Part model, mm, in its own coordinate system. Face numbers are marked on the shaded views. A direction names the side the tool comes from. Round coordinates to 2 decimals unless told otherwise and drop trailing zeros. Write each loop counter-clockwise with the first axis right and the second up, starting at its lowest first coordinate (ties: lowest second). Pieces come first, ordered by that corner, then holes.
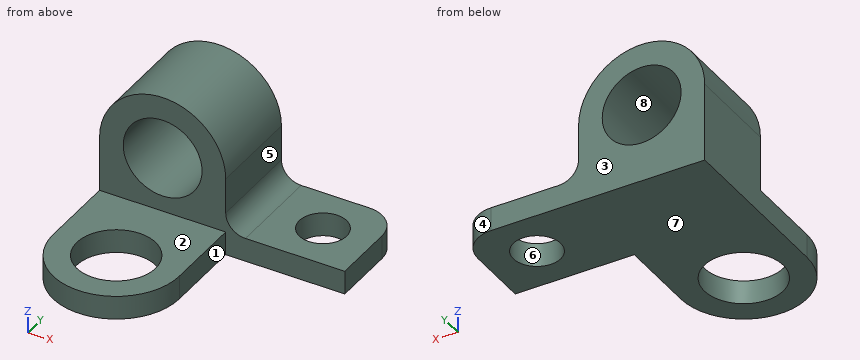
```python
from build123d import *

# Parameters (mm, degrees)
F0_R     = 50
F1_DEPTH = 120
F2_R     = 30
F3_DEPTH = 30
F4_R     = 50
F5_DEPTH = 30


with BuildPart() as f1:
    # F0 (on Front) → F1 (new body)
    with BuildSketch(Plane.XZ):
        with BuildLine():
            Line((0, 100), (0, 0))
            Line((0, 0), (311, 0))
            Line((311, 0), (311, 30))
            Line((311, 30), (185, 30))
            ThreePointArc((185, 30), (167.32233, 37.32233), (160, 55))
            Line((160, 55), (160, 100))
            ThreePointArc((160, 100), (80, 180), (0, 100))
        make_face()
        with Locations((80, 100)):
            Circle(F0_R, mode=Mode.SUBTRACT)
    extrude(amount=F1_DEPTH)

    # F2 (on face) → F3 (cut)
    with BuildSketch(Plane.XY.offset(30)):
        with Locations((248, -60)):
            Circle(F2_R)
        with BuildLine():
            Line((311, 0), (271, 0))
            ThreePointArc((271, 0), (299.284271, -11.715729), (311, -40))
            Line((311, -40), (311, 0))
        make_face()
    extrude(amount=-F3_DEPTH, mode=Mode.SUBTRACT)

    # F4 (on face) → F5 (join)
    with BuildSketch(Plane(origin=(0, 0, 0), x_dir=(1, 0, 0), z_dir=(0, 0, -1))):
        with BuildLine():
            Line((0, 220), (0, 120))
            Line((0, 120), (160, 120))
            Line((160, 120), (160, 220))
            ThreePointArc((160, 220), (80, 300), (0, 220))
        make_face()
        with Locations((80, 220)):
            Circle(F4_R, mode=Mode.SUBTRACT)
    extrude(amount=-F5_DEPTH)


solid = f1.part
```
Q1. Cut at B-B on x = 80. Write the cut outline in (y, z), plus the area to 3 significant figures.
Values follow:
outline: (-300, 0) - (-270, 0) - (-270, 30) - (-300, 30) - close; (-170, 0) - (0, 0) - (0, 50) - (-120, 50) - (-120, 30) - (-170, 30) - close; (-120, 150) - (0, 150) - (0, 180) - (-120, 180) - close
area: 12,000 mm2
Q2. Mould opens along Z. For the marked faces 6, 7 and 8 say: +Z half, -Z half, draft (parallel to the pull), parting line (faces both ways), or undercut.
Values follow:
face 6: draft
face 7: -Z half
face 8: undercut
Q3. Cut at A-A on y = -60. Write the cut outline in (x, z), plus the area to 3 significant figures.
Values follow:
outline: (0, 0) - (218, 0) - (218, 30) - (185, 30) arc R25 cw to (160, 55) - (160, 100) arc R80 ccw to (0, 100) - close; (278, 0) - (311, 0) - (311, 30) - (278, 30) - close; hole circle Ø100 at (80, 100)
area: 21,100 mm2
Q4. Drop flat-ended pins along their axis: pin 1 (10 mm diameter, centred on x = 220, y = -41, fed in from -Z); pin 2 (1.5 mm diameter, centred on y = -58.5, z = 90, fed in from +X); pin 3 (3 mm diameter, centred on x = 33, z = 63, fed in from -Y); pin 4 (6 mm diameter, centred on x = 81, y = -167, fed in from +Z). Give the stop position or say it passes through.
Values follow:
pin 1: stops at z = 0
pin 2: stops at x = 160
pin 3: stops at y = -120
pin 4: stops at z = 30
Q5. Cut at D-D on z = 134. Write the cut outline in (x, y).
Values follow:
outline: (7.58, -120) - (43.34, -120) - (43.34, 0) - (7.58, 0) - close; (116.66, -120) - (152.42, -120) - (152.42, 0) - (116.66, 0) - close
Q6. Cut at C-C on x = 248. Write the cut outline in (y, z), plus the area to 3 significant figures.
Values follow:
outline: (-120, 0) - (-90, 0) - (-90, 30) - (-120, 30) - close; (-30, 0) - (0, 0) - (0, 30) - (-30, 30) - close
area: 1,800 mm2
Q7. Which spindle directions (+Z, -Z, +X, -X, +Y, -Y) get a long thin tool onto all of the face, cutting with end or side? Do the marked faces 1, 2, 3, 4 and 5. Say none if no direction does.
Values follow:
face 1: +Z, -Z, +X, -Y
face 2: +Z, +X, -X, -Y
face 3: +Z, -Z, +X, -X, +Y
face 4: +Z, -Z, +X, +Y
face 5: +Z, +X, +Y, -Y
Q8. Wall check: L1, parallel to Y at x = 80, z = 7; L2, parallel to Y at x = 248, z = 8; L3, parallel to X at y = -220, z = 20.5. Give the ranges that are in metal, low to high.
Values follow:
L1: y = -300 to -270, -170 to 0
L2: y = -120 to -90, -30 to 0
L3: x = 0 to 30, 130 to 160
